Autodesk Fusion 360 part; units mm, degrees
sketch "Sketch1" plane through (0, 0, 0) normal (0, 1, 0) x (1, 0, 0)
  circle A0 centre (0, 0) radius 48 construction
  circle A1 centre (0, 0) radius 14 construction
  circle A2 centre (0, 0) radius 9.5 construction
  circle A3 centre (0, 0) radius 8 construction
  line L0 (0, 0) -> (8, 0) construction
  line L1 (0, 0) -> (0, -9.5) construction
  line L2 (0, 0) -> (-8, 0) construction
  line L3 (0, 0) -> (0, 9.5) construction
  circle A4 centre (8, 0) radius 1.5 construction
  circle A5 centre (-8, 0) radius 1.5 construction
  circle A6 centre (0, 9.5) radius 1.5 construction
  circle A7 centre (0, 0) radius 12 construction
  line L4 (8, 0) -> (18, 0) construction
  line L5 (21.1, 0) -> (19.55, 2.6847) construction
  line L6 (19.55, 2.6847) -> (16.45, 2.6847) construction
  line L7 (16.45, 2.6847) -> (14.9, 0) construction
  line L8 (14.9, 0) -> (16.45, -2.6847) construction
  line L9 (16.45, -2.6847) -> (19.55, -2.6847) construction
  line L10 (19.55, -2.6847) -> (21.1, 0) construction
  circle A8 centre (18, 0) radius 3.1 construction
  circle A9 centre (18, 0) radius 1.5
  line L11 (0, 52) -> (-68, 52) construction
  line L12 (-9.7468, 47) -> (-68, 47) construction
  line L13 (-68, 52) -> (-68, 47) construction
  line L14 (-68, 47) -> (-68, 35.633) construction
  line L15 (-68, 35.633) -> (-32.1604, 35.633) construction
  line L16 (-68, 35.633) -> (-68, 30.833) construction
  line L17 (-68, 30.833) -> (-36.7876, 30.833) construction
  line L18 (-68, 30.833) -> (-68, -9.167) construction
  line L19 (-60, -9.167) -> (-47.1165, -9.167)
  line L20 (-68, -9.167) -> (-68, -13.967) construction
  line L21 (-68, -13.967) -> (-45.923, -13.967) construction
  line L22 (-60, -13.967) -> (-60, 35.633)
  line L23 (5.9333, 10.4305) -> (19.5328, 2.6945)
  line L24 (-60, -13.967) -> (21.1, -13.967)
  line L25 (21.1, -13.967) -> (21.1, 0)
  arc A10 (21.1, 0) -> (19.5328, 2.6945) centre (18, 0) ccw
  line L26 (-60, 35.633) -> (5, 35.633)
  line L27 (5, 35.633) -> (5, 11.8322)
  arc A11 (5.9333, 10.4305) -> (5.7778, 10.5175) centre (0, 0) ccw
  arc A12 (5, 11.8322) -> (5.7778, 10.5175) centre (6.5, 11.8322) ccw
  arc A13 (5.7778, 10.5175) -> (7.9656, 11.513) centre (6.5, 11.8322) ccw construction
  arc A14 (5.4445, 12.898) -> (5, 11.8322) centre (6.5, 11.8322) ccw construction
  arc A15 (7.9656, 11.513) -> (5.4445, 12.898) centre (6.5, 11.8322) ccw construction
  line L28 (5, 11.8322) -> (5, 10.9087) construction
  arc A16 (5.7778, 10.5175) -> (5, 10.9087) centre (0, 0) ccw construction
  line L29 (-60, 30.833) -> (5, 30.833)
  line L30 (-47.1165, -9.167) -> (21.1, -9.167)
  line L31 (-60, 35.633) -> (-60, 45.633)
  line L32 (-60, 45.633) -> (5, 45.633)
  line L33 (5, 45.633) -> (5, 35.633)
  circle A17 centre (-56, 42) radius 1.5
  circle A18 centre (-40, 42) radius 1.5
  line L34 (-40, 42) -> (0, 0) construction
  circle A19 centre (-55.8448, -4.167) radius 1.5
  line L35 (0, 0) -> (-55.8448, -4.167) construction
  line L36 (-68, -9.167) -> (-60, -9.167) construction
  circle A20 centre (0, 0) radius 2.5
  circle A21 centre (0, 0) radius 6
  point P0 (18, 0)
  point P1 (-33.1034, 34.7586)
  point P2 (-47.8669, -3.5717)
  dimension "d1" = 96
  dimension "d2" = 28
  dimension "d3" = 19
  dimension "d4" = 16
  dimension "d5" = 3
  dimension "d6" = 3
  dimension "d7" = 3
  dimension "d8" = 24
  dimension "d9" = 18
  dimension "d10" = 3.1
  dimension "d11" = 60
  dimension "d12" = 3
  dimension "d13" = 52
  dimension "d14" = 68
  dimension "d15" = 68
  dimension "d18" = 5
  dimension "d22" = 16.367
  dimension "d23" = 4.8
  dimension "d24" = 40
  dimension "d25" = 4.8
  dimension "d26" = 8
  dimension "d27" = 3.1
  dimension "d28" = 5
  dimension "d33" = 12
  dimension "d34" = 3
  dimension "d35" = 10
  dimension "d36" = 3
  dimension "d37" = 12
  dimension "d38" = 5
  dimension "d39" = 3
  dimension "d40" = 5
  dimension "d41" = 10
  dimension "d42" = 3
  dimension "d43" = 5
  dimension "d44" = 8
  dimension "d51" = 5
  dimension "d52" = 12
extrude "Extrude1" add sketch "Sketch1" along normal blind 4.8 contours L19 L22 L23 L25 A10 L27 A11 A12 L29 L30 | L19 L22 L24 L25 L30 | L22 L26 L27 L29 | L26 L31 L32 L33 | A21
fillet "Fillet1" radius 4 2 edges at (5, 2.4, -45.633) (-60, 2.4, -45.633)
extrude "Extrude3" cut sketch "Sketch1" along normal blind 3.2 contours A21
sketch "Sketch2" plane through (0, 4.8, 0) normal (0, 1, 0) x (-1, 0, 0)
  arc A0 (56, -45.633) -> (60, -41.633) centre (56, -41.633) ccw
  line L0 (60, -41.633) -> (60, 13.967)
  line L1 (60, 13.967) -> (-21.1, 13.967)
  line L2 (-21.1, 13.967) -> (-21.1, 0)
  arc A1 (-21.1, 0) -> (-19.5328, -2.6945) centre (-18, 0) ccw
  line L3 (-19.5328, -2.6945) -> (-5.9333, -10.4305)
  arc A2 (-5.9333, -10.4305) -> (-5.7778, -10.5175) centre (0, 0) ccw
  arc A3 (-5, -11.8322) -> (-5.7778, -10.5175) centre (-6.5, -11.8322) ccw
  line L4 (-5, -11.8322) -> (-5, -41.633)
  arc A4 (-5, -41.633) -> (-1, -45.633) centre (-1, -41.633) ccw
  line L5 (-1, -45.633) -> (56, -45.633)
  circle A5 centre (0, 0) radius 2.5
  circle A6 centre (55.8448, 4.167) radius 1.5
  circle A7 centre (40, -42) radius 1.5
  circle A8 centre (56, -42) radius 1.5
  circle A9 centre (-18, 0) radius 1.5
  line L6 (47.1165, 9.167) -> (-21.1, 9.167)
  line L7 (60, 9.167) -> (47.1165, 9.167)
  line L8 (60, -30.833) -> (-5, -30.833)
  line L9 (60, -35.633) -> (-5, -35.633)
  line L10 (-21.1, 13.967) -> (60, 13.967)
  line L11 (60, 13.967) -> (60, 9.167)
  line L12 (60, 9.167) -> (-21.1, 9.167)
  line L13 (-21.1, 9.167) -> (-21.1, 13.967)
  line L14 (-5, -30.833) -> (60, -30.833)
  line L15 (60, -30.833) -> (60, -35.633)
  line L16 (60, -35.633) -> (-5, -35.633)
  line L17 (-5, -35.633) -> (-5, -30.833)
extrude "Extrude4" cut sketch "Sketch2" against normal blind 1.8 contours L0 L4 L8 L9 L14 L15 L16 L17 | L0 L1 L2 L6 L7 L10 L11 L12 L13
Can you work these out from the model? Positions are in its coordinate system, mm. A direction names the side the tool comes from. Give positions to 0.01 mm unless a question says otherwise; leave off trailing zeros. Loops run counter-clockwise (first coordinate to the right, second up) from the corner with the lowest first, then second, coordinate; pieces in that order, holes last. Notation, with made-up numbers: (42.5, -17.75) -> (89.5, -17.75) arc R18 ccw to (89.5, -2.75) -> close; hole circle Ø3 at (78, 42.25). An arc over 180 degrees is marked (long way). Use one line per item in the form item = value.
1) If we section it at B-B (y = 4.05): Please give me the cut outline in (x, z).
Answers:
outline = (-60, -41.63) arc R4 ccw to (-56, -45.63) -> (1, -45.63) arc R4 ccw to (5, -41.63) -> (5, -35.63) -> (-60, -35.63) -> close; (-60, -30.83) -> (5, -30.83) -> (5, -11.83) arc R1.5 cw to (5.78, -10.52) arc R12 ccw to (5.93, -10.43) -> (19.53, -2.69) arc R3.1 ccw to (21.1, 0) -> (21.1, 9.17) -> (-60, 9.17) -> close; hole circle Ø3 at (-56, -42); hole circle Ø3 at (-55.84, 4.17); hole circle Ø3 at (-40, -42); hole circle Ø5 at (0, 0); hole circle Ø3 at (18, 0)
2) I need wall thicknesses on line 1 along X through (y, z) = (4.05, 0); line 2 along X through (y, z) = (2.15, 0); line 3 along Z through (x, y) = (-56, 2.55). Which ranges of each line are inside material? Lowest first, please.
Answers:
line_1 = -60 to -2.5, 2.5 to 16.5, 19.5 to 21.1
line_2 = -60 to -6, 6 to 16.5, 19.5 to 21.1
line_3 = -45.63 to -43.5, -40.5 to 2.68, 5.66 to 13.97
3) We'd pull the mould along X, two halves only. Please class faces 1 (the face through (-27, 3, -33)), 2 (the face through (-55.31, 2.37, -43.33)), 3 (the face through (12.638, 2.366, -6.617)): released by +X, released by -X, zero draft, split by the parting line, or undercut.
Answers:
face_1 = zero draft
face_2 = undercut
face_3 = released by +X
4) If we section it at C-C (x = -45): Please give me the cut outline in (y, z).
Answers:
outline = (0, -45.63) -> (4.8, -45.63) -> (4.8, -35.63) -> (3, -35.63) -> (3, -30.83) -> (4.8, -30.83) -> (4.8, 9.17) -> (3, 9.17) -> (3, 13.97) -> (0, 13.97) -> close
5) For faces 4 (the face through (-28, 4, -35.633)), 5 (the face through (-19, 3, 12)), 6 (the face through (-29, 4.8, -11)), which set-ups out of +Z, -Z, +X, -X, +Y, -Y let a thin tool reach every point of the face, with its end or its side?
Answers:
face_4 = +X, -X, +Y
face_5 = +Z, +X, -X, +Y
face_6 = +Z, -Z, +X, -X, +Y
6) If we section it at D-D (z = -18.5): Please give me the cut outline in (x, y), plus the area to 3 significant figures.
Answers:
outline = (-60, 0) -> (5, 0) -> (5, 4.8) -> (-60, 4.8) -> close
area = 312 mm²
7) If we section it at A-A (x = 0): Please give me the cut outline in (y, z), plus the area to 3 significant figures.
Answers:
outline = (0, -45.63) -> (4.8, -45.63) -> (4.8, -35.63) -> (3, -35.63) -> (3, -30.83) -> (4.8, -30.83) -> (4.8, -2.5) -> (3.2, -2.5) -> (3.2, -6) -> (0, -6) -> close; (0, 6) -> (3.2, 6) -> (3.2, 2.5) -> (4.8, 2.5) -> (4.8, 9.17) -> (3, 9.17) -> (3, 13.97) -> (0, 13.97) -> close
area = 222 mm²
8) Will these pins go through, and if not, where does the flat tip stop? pin 1 (1.4 mm diameter, centred on x = -16, z = -34.5, fed in from +Y); pin 2 (0.9 mm diameter, centred on x = -25.5, y = 4, fed in from +Z); pin 3 (2.5 mm diameter, centred on x = -55.84, z = 4.17, fed in from -Y).
Answers:
pin_1 = 3
pin_2 = 9.17
pin_3 = through
